Autodesk Inventor part; units mm, degrees
ref_plane "YZ Plane" through (0, 0, 0) normal (1, 0, 0) x (0, 1, 0)
ref_plane "XZ Plane" through (0, 0, 0) normal (0, 1, 0) x (-1, 0, 0)
ref_plane "XY Plane" through (0, 0, 0) normal (0, 0, 1) x (1, 0, 0)
sketch "Sketch1" plane through (0, 0, 0) normal (0, 1, 0) x (-1, 0, 0)
  circle A0 centre (0, 0) radius 14.5
  line L0 (0, 0) -> (14.5, 0)
  line L1 (0, 0) -> (0, 14.5)
  dimension "d0" = 29
extrude "Extrusion1" add sketch "Sketch1" along normal blind 8 contours L0 L1 A0 picked at (1.0755, 9.5455)
sketch "Sketch2" plane through (0, 8, 0) normal (0, 1, 0) x (1, 0, 0)
  line L0 (0, -14.5) -> (0, 0)
  circle A0 centre (0, 0) radius 2.375
  circle A1 centre (0, 0) radius 3.5
  arc A2 (-14.5, 0) -> (0, -14.5) centre (0, 0) ccw
  line L1 (0, -14.5) -> (3.3965, -0.8448)
  line L2 (0, 0) -> (-14.5, 0)
  line L3 (-14.5, 0) -> (-0.8448, 3.3965)
  point P0 (-2.375, 0)
  point P1 (0, -2.375)
  dimension "d3" = 4.75
  dimension "d4" = 7
extrude "Extrusion2" add sketch "Sketch2" against normal blind 8 contours L0 A1 L1 | L0 A0 L2 A1 | L3 A1 L2 picked at (3.0951, 0.2624)
sketch "Sketch3" plane through (0, 8, 0) normal (0, 1, 0) x (1, 0, 0)
  line L0 (0, 0) -> (-2.375, 0)
  circle A0 centre (0, 0) radius 2.375
extrude "Extrusion3" cut sketch "Sketch3" against normal blind 8
sketch "Sketch4" plane through (0, 8, 0) normal (0, 1, 0) x (1, 0, 0)
  arc A0 (-14.5, 0) -> (0, -14.5) centre (0, 0) ccw
  line L0 (-14.5, 0) -> (-0.8448, 3.3965)
  line L1 (0, -14.5) -> (-14.5, 0)
  line L2 (-14.5, 0) -> (-23.5148, -10.1914)
  line L3 (-23.5148, -10.1914) -> (-2.2293, -23.4627)
  line L4 (3.3965, -0.8448) -> (0, -14.5)
  line L5 (-2.2293, -23.4627) -> (0, -14.5)
extrude "Extrusion4" cut sketch "Sketch4" against normal blind 10 contours L1 A0
properties part number "bell_crank_v2"
Geometry check sheet. Reference: the model listing, model coordinates, mm. Round coordinates to 2 decimals unless told otherwise and drop trailing zeros. Order: outer loops, then holes, each group sorted by start corner. A loop starts at its lowest first (then second) coordinate and runs counter-clockwise, first axis right, second up. Notation, with made-up numbers: (56.5, 31) - (85.5, 31) arc R25 cw to (85.5, 43) - close; hole circle Ø1 at (-37, 20). An arc over 180 degrees is marked (long way). Use a Markdown table: item, result. Add a question column.
1) Section check A-A (x = 0.75). Record the cut outline in (y, z), then the cut area to 3 significant figures.
2) Mould release check, pull along X, two halves, no side actions. Record for faces 1 (the flat face through (1.674, 4.056, 7.768)), 2 (the cylindrical face through (0.51, 4.06, -2.32)), 3 (the flat face through (-7.1, 4.1, 7.4)): released by +X, released by -X, zero draft, split by the parting line, or undercut.
3) Section check B-B (z = 1.75). Record the cut outline in (x, y).
4) Gauge pin test, flat ends, axial feed: P1, Ø1, axis at y = 1, z = 7.5, coming from the -X side; P2, Ø5.5, axis at x = 0, z = 0, coming from the +Y side; P3, Ø1.5, axis at y = 1, z = 5.5, coming from the -X side; P4, Ø3, axis at y = 2, z = 0.5, coming from the -X side. Record the tip position at first contact, or that the pin passes through.
5) Section check D-D (x = -6.25). Record the cut outline in (y, z).
6) Thickness scan on line 1 along X through (y, z) = (3, 0.5); line 2 along Z through (x, y) = (-5.25, 0.5); line 3 along Z through (x, y) = (-7.5, 3.75). Record the ranges inside material, lowest first.
Established:
| question | item | result |
|---|---|---|
| 1 | outline | (0, -3.42) - (8, -3.42) - (8, -2.25) - (0, -2.25) - close; (0, 2.25) - (8, 2.25) - (8, 11.48) - (0, 11.48) - close |
| 1 | area | 83.2 mm2 |
| 2 | face 1 | released by +X |
| 2 | face 2 | undercut |
| 2 | face 3 | released by -X |
| 3 | outline | (-12.75, 0) - (-1.61, 0) - (-1.61, 8) - (-12.75, 8) - close; (1.61, 0) - (3.17, 0) - (3.17, 8) - (1.61, 8) - close |
| 4 | P1 | x = -7.5 |
| 4 | P2 | y = 8 |
| 4 | P3 | x = -9.75 |
| 4 | P4 | x = -14.5 |
| 5 | outline | (0, -2.05) - (8, -2.05) - (8, 8.25) - (0, 8.25) - close |
| 6 | line 1 | -14 to -2.32, 2.32 to 3.46 |
| 6 | line 2 | -2.3 to 9.25 |
| 6 | line 3 | -1.74 to 7 |
